Design review of the part built by this model. Coordinates are the model's own, in mm. A direction names the side the tool comes from. Coordinates: 2 decimals unless noted, no trailing zeros. Write each loop counter-clockwise with the first axis right and the second up, starting at its lowest first coordinate (ties: lowest second). Pieces come first, ordered by that corner, then holes.
Q1. For probe 1 along Y at (x, z) = (4, 6); probe 2 along Z at (x, y) = (11.5, 22); probe 3 along Z at (x, y) = (5, 13), list the stretches that pass through material, from the lowest coordinate up.
Q2. Insertion check: pin 1 (6 mm diameter, centred on x = 10, y = 8, fed in from +Z); pin 2 (4 mm diameter, centred on y = 18, z = 8, fed in from +X); pin 3 (1.5 mm diameter, centred on y = 23.5, z = 9, fed in from -X); pin 4 (1.5 mm diameter, centred on x = 4, z = 7.5, fed in from +Y). Each pin has a flat end and moves straight along its axis. Give the tip position at first contact, or say it passes through.
Q3. Take a section at C-C (z = 5.5). Give the boundary of the cut face in (x, y).
Q4. Take a section at B-B (x = 2.75). Give the boundary of the cut face in (y, z), and give its area (3 significant figures).
Q5. Take a section at D-D (x = 18.25). Give the boundary of the cut face in (y, z), and give its area (3 significant figures).
Q6. Machinability: for faces 1 (the flat face through (3.585, 14.902, 6.272)), 2 (the flat face through (10, 0, 1)), 3 (the flat face through (5, 22, 5)), 4 (the flat face through (5, 8, 5)), 5 (the flat face through (7.713, 15, 6)), which of the approach directions +Z, -Z, +X, -X, +Y, -Y give a long, thin tool a straight path to every point of the face, cutting with its end or side? Answer none if there is none.
Q7. Take a section at A-A (y = 20.25). Give the boundary of the cut face in (x, z).
```python
from build123d import *

# Parameters (mm, degrees)
F0_W     = 20
F0_H     = 30
F1_DEPTH = 2
F3_START = -8
F3_DEPTH = 14
F4_SIZE  = 1


with BuildPart() as f1:
    # F0 (on Top) → F1 (new body)
    with BuildSketch(Plane.XY):
        with Locations((10, 15)):
            Rectangle(F0_W, F0_H)
    extrude(amount=F1_DEPTH)

    # F2 (on face) → F3 (join)
    with BuildSketch(Plane.XZ.offset(F3_START)):
        Polygon((7.7134513162, 11.1925333174), (0, 2), (7.7134513162, 2), align=None)
    extrude(amount=-F3_DEPTH)

    # F4
    f4_edges = [f1.edges().sort_by_distance(p)[0] for p in [
        (7.713451, 15, 11.192533),
    ]]
    chamfer(f4_edges, length=F4_SIZE)


solid = f1.part
```
Response:
1. probe 1: y = 8 to 22
1. probe 2: z = 0 to 2
1. probe 3: z = 0 to 7.96
2. pin 1: stops at z = 10.43
2. pin 2: stops at x = 7.71
2. pin 3: passes through
2. pin 4: stops at y = 22
3. outline: (2.94, 8) - (7.71, 8) - (7.71, 22) - (2.94, 22) - close
4. outline: (0, 0) - (30, 0) - (30, 2) - (22, 2) - (22, 5.28) - (8, 5.28) - (8, 2) - (0, 2) - close
4. area: 106 mm2
5. outline: (0, 0) - (30, 0) - (30, 2) - (0, 2) - close
5. area: 60.0 mm2
6. face 1: +Z, -X, +Y, -Y
6. face 2: +Z, -Z, +X, -X, -Y
6. face 3: +Z, +X, -X, +Y
6. face 4: +Z, +X, -X, -Y
6. face 5: +Z, +X, +Y, -Y
7. outline: (0, 0) - (20, 0) - (20, 2) - (7.71, 2) - (7.71, 10.19) - (7.07, 10.43) - (0, 2) - close
